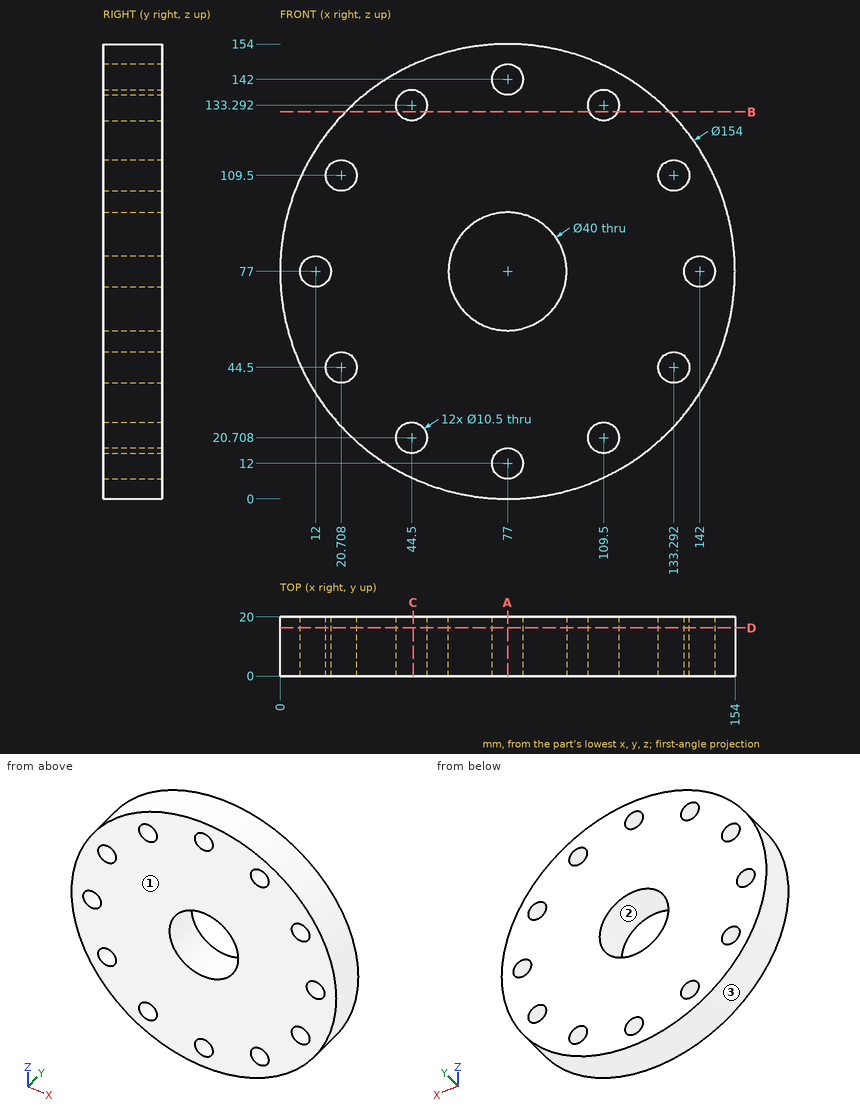
Input: dimensioned drawing with shaded views. Units: mm. Origin: part minimum x, y, z. Coordinates: 2 decimals unless noted, no trailing zeros. Order: outer loops, then holes, each group sorted by start corner. A loop starts at its lowest first (then second) coordinate and runs counter-clockwise, first axis right, second up.
Item 1: Draft query along Z for the marked faces 1, 2 and 3. Return one class per face: released by +Z, released by -Z, zero draft, split by the parting line, or undercut.
Answer:
face 1: zero draft
face 2: undercut
face 3: split by the parting line
Item 2: Section query A-A (x = 77). Output: boundary loops of the cut face in (y, z), then the cut area to 3 significant figures.
Answer:
outline: (0, 0) - (20, 0) - (20, 6.75) - (0, 6.75) - close; (0, 17.25) - (20, 17.25) - (20, 57) - (0, 57) - close; (0, 97) - (20, 97) - (20, 136.75) - (0, 136.75) - close; (0, 147.25) - (20, 147.25) - (20, 154) - (0, 154) - close
area: 1,860 mm2
Item 3: Section query D-D (y = 16.25). State how many separate pieces and enclosed holes the cut face has, then the cut area to 3 significant figures.
Answer:
separate pieces: 1
enclosed holes: 13
area: 16,300 mm2
Item 4: Section query B-B (z = 131). Output: boundary loops of the cut face in (x, y), then the cut area to 3 significant figures.
Answer:
outline: (22.11, 0) - (39.78, 0) - (39.78, 20) - (22.11, 20) - close; (49.22, 0) - (104.78, 0) - (104.78, 20) - (49.22, 20) - close; (114.22, 0) - (131.89, 0) - (131.89, 20) - (114.22, 20) - close
area: 1,820 mm2
Item 5: Material intervals for line 1 along Z through (x, y) = (25, 5.75) (1 decimal); line 2 along Z through (x, y) = (109, 1.5) (1 decimal); line 3 along X through (y, z) = (19.25, 76) (1 decimal), sorted ascending.
Answer:
line 1: z = 20.2 to 41.5, 47.5 to 106.5, 112.5 to 133.8
line 2: z = 7 to 15.5, 25.9 to 128.1, 138.5 to 147
line 3: x = 0 to 6.8, 17.2 to 57, 97 to 136.8, 147.2 to 154
Item 6: Section query C-C (x = 45). Output: boundary loops of the cut face in (y, z) (1 decimal), then the cut area to 3 significant figures.
Answer:
outline: (0, 7) - (20, 7) - (20, 15.5) - (0, 15.5) - close; (0, 25.9) - (20, 25.9) - (20, 128.1) - (0, 128.1) - close; (0, 138.5) - (20, 138.5) - (20, 147) - (0, 147) - close
area: 2,380 mm2
Item 7: Contact query for flat-ended pins moving along their axis: P1, Ø6, axis at y = 3, z = 86.5, coming from the +X side (1 decimal); P2, Ø3, axis at x = 82, y = 16.5, coming from the +Z side; P3, Ø1, axis at y = 4.5, z = 48.5, coming from the -X side. Output: stop coordinate, or through.
Answer:
P1: stops at x = 153.7
P2: stops at z = 153.92
P3: stops at x = 5.27
